```python
from build123d import *

# Parameters (mm, degrees)
SKETCH1_W           = 9.5
SKETCH1_H           = 3.5
SKETCH1_W_2         = 2.5
BOSS_EXTRUDE1_DEPTH = 10
CHAMFER1_SIZE       = 3
CHAMFER2_SIZE       = 1.2
SKETCH2_R           = 1.6
CUT_EXTRUDE1_DEPTH  = 10


with BuildPart() as part:
    # Sketch1 → Boss-Extrude1 (new body)
    with BuildSketch(Plane.XY):
        with Locations((25.25, 3.25)):
            Rectangle(SKETCH1_W, SKETCH1_H)
        Polygon((20.5, 15.5), (-20.5, 15.5), (-20.5, -15.5), (20.5, -15.5), (20.5, -5), (18, -5), (18, -13), (-18, -13), (-18, 13), (18, 13), (18, 5), (20.5, 5), align=None)
        with Locations((19.25, -3.25)):
            Rectangle(SKETCH1_W_2, SKETCH1_H)
        with Locations((19.25, 3.25)):
            Rectangle(SKETCH1_W_2, SKETCH1_H)
        with Locations((25.25, -3.25)):
            Rectangle(SKETCH1_W, SKETCH1_H)
    extrude(amount=BOSS_EXTRUDE1_DEPTH)

    # Chamfer1
    chamfer1_edges = [part.edges().sort_by_distance(p)[0] for p in [
        (20.5, -5, 5),
        (20.5, 5, 5),
    ]]
    chamfer(chamfer1_edges, length=CHAMFER1_SIZE)

    # Chamfer2
    chamfer2_edges = [part.edges().sort_by_distance(p)[0] for p in [
        (30, 5, 5),
        (30, 1.5, 5),
        (18, 1.5, 5),
        (18, 13, 5),
        (-18, 13, 5),
        (-18, -13, 5),
        (18, -13, 5),
        (18, -1.5, 5),
        (30, -1.5, 5),
        (30, -5, 5),
        (20.5, -15.5, 5),
        (-20.5, -15.5, 5),
        (-20.5, 15.5, 5),
        (20.5, 15.5, 5),
    ]]
    chamfer(chamfer2_edges, length=CHAMFER2_SIZE)

    # Sketch2 → Cut-Extrude1 (cut)
    with BuildSketch(Plane(origin=(0, 5, 0), x_dir=(1, 0, 0), z_dir=(0, 1, 0))):
        with Locations(Location((25.8, -5, 0), (0, 0, 180))):
            Circle(SKETCH2_R)
    extrude(amount=-CUT_EXTRUDE1_DEPTH, mode=Mode.SUBTRACT)


solid = part.part
```
Can you work these out from the model? Positions are in its coordinate system, mm. A direction names the side the tool comes from. Coordinates: 2 decimals unless noted, no trailing zeros. Write each loop counter-clockwise with the first axis right and the second up, starting at its lowest first coordinate (ties: lowest second). Pieces come first, ordered by that corner, then holes. Notation, with made-up numbers: M 8,83.5 L 36,83.5 A15 cw 36,107.5 Z; hole C 50,76 d1. An arc over 180 degrees is marked long. Write item = value, one per line. Start each with the question number.
Q1. If we section it at D-D, the plane z = 5: State how many separate pieces and enclosed holes the cut face has, then the cut area to 3 significant figures.
Q2. If we section it at A-A, the plane y = 4.5: Write out the boundary of the cut face in (x, z).
Q3. If we section it at C-C, the plane y = -12.5: Write out the boundary of the cut face in (x, z).
Q4. Thinking about a two-plate mould opening in Z: for faces 1 (the face through (30, -3, 5)), 2 (the face through (24.32, -3.23, 4.39)), which applies, released by +Z, released by -Z, zero draft, split by the parting line, or undercut?
Q5. If I drill on L1, parallel to Y at x = -3, z = 1; L2, parallel to Z at x = 25.8, y = 3.4; L3, parallel to X at y = -3.5, z = 7.5, over which ranges is the centre line in solid material (lowest first)? Write a range as [from, to].
Q6. On a 3-axis mill with a long thin cutter (end or side, diameter ignored), from which of +Z, -Z, +X, -X, +Y, -Y can I reach the whole of each face in a straight line? I mean faces 3 (the face through (27.3, 5, 3.8)), 4 (the face through (24, -1.5, 5)), 5 (the face through (24.32, 3.27, 4.39)), 6 (the face through (27.3, -5, 3.8)), 7 (the face through (-18, 0, 5)). Say none if no direction works.
Q7. If we section it at B-B, the plane x = 22.5: Write out the boundary of the cut face in (y, z).
Q8. I'm going to push flat-ended pins straight in: pin 1 (2.5 mm diameter, centred on x = 26, z = 7, fed in from -Y); pin 2 (3 mm diameter, centred on x = 25.8, z = 5, fed in from -Y); pin 3 (5 mm diameter, centred on y = 12, z = 3.5, fed in from +X); pin 4 (3.5 mm diameter, centred on x = 25.8, z = 5, fed in from +Y). Where does each tip first touch, or does it pass through?
Check sheet entries:
q1.separate_pieces = 3
q1.enclosed_holes = 0
q1.area = 376 mm²
q2.outline = M -20.5,0 L -18,0 L -18,10 L -20.5,10 Z; M 18,0 L 29.3,0 L 29.3,10 L 18,10 Z; hole C 25.8,5 d3.2
q3.outline = M -20.5,0 L -17.3,0 L -17.3,10 L -20.5,10 Z; M 17.3,0 L 20.5,0 L 20.5,10 L 17.3,10 Z
q4.face_1 = zero draft
q4.face_2 = undercut
q5.L1 = [-15.5, -13], [13, 15.5]
q5.L2 = [0, 3.4], [6.6, 10]
q5.L3 = [-20.5, -18], [18, 30]
q6.face_3 = +Z, -Z, +X, +Y
q6.face_4 = +Z, -Z, +X
q6.face_5 = +Y, -Y
q6.face_6 = +Z, -Z, +X, -Y
q6.face_7 = +Z, -Z
q7.outline = M -6,0 L -1.5,0 L -1.5,10 L -6,10 Z; M 1.5,0 L 6,0 L 6,10 L 1.5,10 Z
q8.pin_1 = -5
q8.pin_2 = through
q8.pin_3 = 20.5
q8.pin_4 = 5
